Geometry check sheet. Reference: the model listing, model coordinates, mm. Face numbers are marked on the shaded views. A direction names the side the tool comes from. Coordinates: 2 decimals unless noted, no trailing zeros. Write each loop counter-clockwise with the first axis right and the second up, starting at its lowest first coordinate (ties: lowest second). Pieces come first, ordered by that corner, then holes. Notation, with made-up numbers: (-7, 62.5) -> (3, 62.5) arc R20 ccw to (3, 71.5) -> close; hole circle Ø3 at (-7, -18). An arc over 180 degrees is marked (long way). Use a Markdown table: item, result.
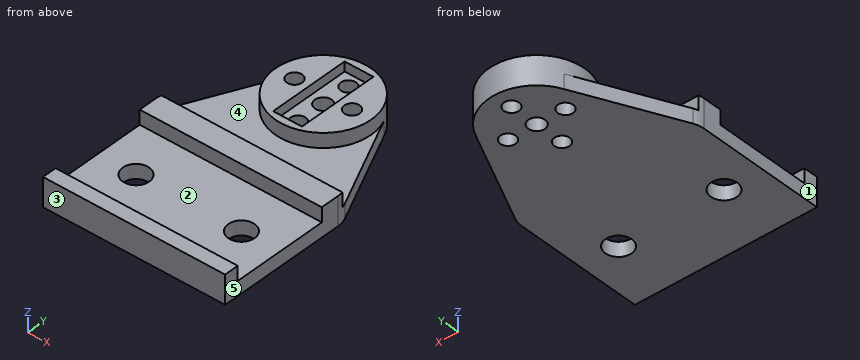
Autodesk Inventor part; units mm, degrees
ref_plane "YZ Plane" through (0, 0, 0) normal (1, 0, 0) x (0, 1, 0)
ref_plane "XZ Plane" through (0, 0, 0) normal (0, 1, 0) x (-1, 0, 0)
ref_plane "XY Plane" through (0, 0, 0) normal (0, 0, 1) x (1, 0, 0)
sketch "スケッチ1" plane through (0, 0, 0) normal (0, 0, 1) x (1, 0, 0)
  line L0 (0, 0) -> (38, 0)
  line L1 (38, 0) -> (38, 28)
  line L2 (0, 28) -> (0, 0)
  circle A0 centre (19, 45) radius 10
  line L3 (19, 45) -> (19, 0)
  line L4 (9, 45) -> (29, 45)
  line L5 (10.069714, 49.5) -> (27.930286, 49.5)
  line L6 (10.069714, 49.5) -> (0, 28)
  line L7 (27.930286, 49.5) -> (38, 28)
  point P0 (28.174131, 48.979363)
  point P1 (9.825869, 48.979363)
  dimension "d0" = 38
  dimension "d1" = 28
  dimension "d3" = 20
  dimension "d56" = 45
  dimension "d71" = 28
  dimension "d73" = 4.5
sketch "スケッチ1 outline for 押し出し1" plane through (0, 0, 0) normal (0, 0, 1) x (1, 0, 0)
  line L0 (9.825869, 48.979363) -> (0, 28)
  line L1 (0, 28) -> (0, 0)
  line L2 (0, 0) -> (38, 0)
  line L3 (38, 0) -> (38, 28)
  line L4 (38, 28) -> (28.174131, 48.979363)
  arc A0 (28.174131, 48.979363) -> (9.825869, 48.979363) centre (19, 45) ccw
extrude "押し出し1" add sketch "スケッチ1 outline for 押し出し1" along normal blind 3
sketch "スケッチ7" plane through (0, 0, 3) normal (0, 0, 1) x (1, 0, 0)
  line L0 (0, 0) -> (38, 0)
  line L1 (38, 0) -> (38, 28)
  line L2 (0, 0) -> (38, 0)
  line L3 (38, 0) -> (38, 3)
  line L4 (38, 3) -> (0, 3)
  line L5 (0, 3) -> (0, 0)
  arc A0 (28.174131, 48.979363) -> (9.825869, 48.979363) centre (19, 45) ccw
  circle A1 centre (19, 45) radius 10
  line L6 (0, 28) -> (0, 0)
  line L7 (0, 28) -> (38, 28)
  line L8 (38, 28) -> (38, 23)
  line L9 (38, 23) -> (0, 23)
  line L10 (0, 23) -> (0, 28)
  point P0 (27.930286, 47.5)
  point P1 (10.069714, 47.5)
  point P2 (0, 23)
  point P3 (29, 43)
  point P4 (9, 43)
  point P5 (10.069714, 47.5)
  point P6 (27.930286, 47.5)
  point P7 (9.486338, 51.080624)
  point P8 (28.513662, 51.080624)
  dimension "d58" = 3
  dimension "d68" = 20
  dimension "d69" = 20
  dimension "d70" = 5
extrude "押し出し4" add sketch "スケッチ7" along normal blind 3 contours L5 L4 L1 L0 | L6 L7 L1 L9 | A1 A0
sketch "スケッチ10" plane through (19, 45, 6) normal (0, 0, 1) x (1, 0, 0)
  line L0 (-3, 8.5) -> (3, 8.5)
  line L1 (3, 8.5) -> (3, -8.5)
  line L2 (3, -8.5) -> (-3, -8.5)
  line L3 (-3, -8.5) -> (-3, 8.5)
  circle A0 centre (0, 0) radius 10
  point P0 (-19, -45)
  dimension "d74" = 8.5
  dimension "d75" = 17
  dimension "d76" = 6
  dimension "d77" = 3
extrude "押し出し7" cut sketch "スケッチ10" against normal blind 2 contours L0 L1 L2 L3
sketch "スケッチ11" plane through (0, 0, 0) normal (0, 0, -1) x (-1, 0, 0)
  arc A0 (-9.825869, 48.979363) -> (-28.174131, 48.979363) centre (-19, 45) ccw
  point P0 (0, 0)
  point P1 (-27.930286, 47.5)
  point P2 (-10.069714, 47.5)
  point P3 (-19, 51)
  point P4 (-25, 45)
  point P5 (-19, 39)
  point P6 (-13, 45)
  dimension "d80" = 6
  dimension "d83" = 360
hole "穴4" at (19, 51, 0) at (25, 45, 0) at (19, 39, 0) at (13, 45, 0) direction (0, 0, 1) diameter 3.2 end through all
sketch "スケッチ12" plane through (0, 0, 0) normal (0, 0, -1) x (-1, 0, 0)
  circle A0 centre (-19, 45) radius 10
  point P0 (0, 0)
hole "穴5" at (19, 45, 0) direction (0, 0, 1) diameter 3.5 end through all
sketch "スケッチ13" plane through (0, 0, 0) normal (0, 0, -1) x (-1, 0, 0)
  circle A0 centre (-19, 45) radius 1.75
  circle A1 centre (-13, 45) radius 1.6
  circle A2 centre (-19, 39) radius 1.6
  circle A3 centre (-25, 45) radius 1.6
  circle A4 centre (-19, 51) radius 1.6
  arc A5 (-9.825869, 48.979363) -> (-28.174131, 48.979363) centre (-19, 45) ccw
  line L0 (-38, 28) -> (-28.174131, 48.979363)
  line L1 (-38, 0) -> (-38, 28)
  line L2 (0, 0) -> (-38, 0)
  line L3 (0, 28) -> (0, 0)
  line L4 (-9.825869, 48.979363) -> (0, 28)
fillet "フィレット1" radius 5 2 edges at (0, 28, 1.5) (38, 28, 1.5)
sketch "スケッチ14" plane through (0, 0, 3) normal (0, 0, 1) x (1, 0, 0)
  line L0 (0, 0) -> (38, 0)
  line L1 (0, 23) -> (0, 3)
  line L2 (38, 3) -> (38, 23)
  point P0 (8, 13)
  point P1 (30, 13)
  dimension "d100" = 13
  dimension "d101" = 13
  dimension "d102" = 8
  dimension "d103" = 8
hole "穴6" at (8, 13, 3) at (30, 13, 3) direction (0, 0, -1) diameter 5.5 end through all
properties part number "robot-arm-frame-base"
Item 1: Section check D-D on x = 19. Record the boundary of the cut face in (y, z), then the cut area to 3 significant figures.
Answer block:
| item | result |
|---|---|
| outline | (0, 0) -> (37.4, 0) -> (37.4, 4) -> (36.5, 4) -> (36.5, 6) -> (35, 6) -> (35, 3) -> (28, 3) -> (28, 6) -> (23, 6) -> (23, 3) -> (3, 3) -> (3, 6) -> (0, 6) -> close; (40.6, 0) -> (43.25, 0) -> (43.25, 4) -> (40.6, 4) -> close; (46.75, 0) -> (49.4, 0) -> (49.4, 4) -> (46.75, 4) -> close; (52.6, 0) -> (55, 0) -> (55, 6) -> (53.5, 6) -> (53.5, 4) -> (52.6, 4) -> close |
| area | 175 mm^2 |
Item 2: Section check C-C on z = 2. Record the boundary of the cut face in (x, y), then the cut area to 3 significant figures.
Answer block:
| item | result |
|---|---|
| outline | (0, 0) -> (38, 0) -> (38, 26.89) arc R5 ccw to (37.53, 29.01) -> (28.17, 48.98) arc R10 ccw to (9.83, 48.98) -> (0.47, 29.01) arc R5 ccw to (0, 26.89) -> close; hole circle Ø5.5 at (8, 13); hole circle Ø3.2 at (13, 45); hole circle Ø3.5 at (19, 45); hole circle Ø3.2 at (19, 39); hole circle Ø3.2 at (19, 51); hole circle Ø3.2 at (25, 45); hole circle Ø5.5 at (30, 13) |
| area | 1,650 mm^2 |
Item 3: Section check A-A on y = 51. Record the boundary of the cut face in (x, z).
Answer block:
| item | result |
|---|---|
| outline | (11, 0) -> (17.4, 0) -> (17.4, 4) -> (16, 4) -> (16, 6) -> (11, 6) -> close; (20.6, 0) -> (27, 0) -> (27, 6) -> (22, 6) -> (22, 4) -> (20.6, 4) -> close |
Item 4: Tool access check on the marked faces 4 and 5. Record the directions out of +Z, -Z, +X, -X, +Y, -Y that give a thin tool (end or side, any length) a straight path to the whole face; none if there is none.
Answer block:
| item | result |
|---|---|
| face 4 | +Z |
| face 5 | +Z, -Z, +X, +Y, -Y |
Item 5: Depth check by flat-ended pin: P1, Ø3.5, axis at x = 19, y = 39, coming from the -Z side; P2, Ø3, axis at x = 33, y = 31, coming from the +Z side; P3, Ø1.5, axis at x = 15.5, z = 5, coming from the +Y side; P4, Ø2.5, axis at x = 27.5, z = 4, coming from the +Y side. Enter the tip coordinate at first touch or a pass-through.
Answer block:
| item | result |
|---|---|
| P1 | stops at z = 0 |
| P2 | stops at z = 3 |
| P3 | stops at y = 54.61 |
| P4 | stops at y = 51.89 |
Item 6: Thickness scan on L1, parallel to X at y = 13, z = 0.9; L2, parallel to Y at x = 19, z = 0.8; L3, parallel to X at y = 45, z = 3.05. Record the ranges inside material, lowest first. Write a range as [from, to].
Answer block:
| item | result |
|---|---|
| L1 | x = [0, 5.25], [10.75, 27.25], [32.75, 38] |
| L2 | y = [0, 37.4], [40.6, 43.25], [46.75, 49.4], [52.6, 55] |
| L3 | x = [9, 11.4], [14.6, 17.25], [20.75, 23.4], [26.6, 29] |
Item 7: Mould release check, pull along Y, two halves, no side actions. Record for the marked faces 1, 2 and 3: +Y half, -Y half, draft (parallel to the pull), parting line (faces both ways), or undercut.
Answer block:
| item | result |
|---|---|
| face 1 | draft |
| face 2 | undercut |
| face 3 | -Y half |
Item 8: Section check B-B on x = 13. Record the boundary of the cut face in (y, z).
Answer block:
| item | result |
|---|---|
| outline | (0, 0) -> (43.4, 0) -> (43.4, 6) -> (37, 6) -> (37, 3) -> (28, 3) -> (28, 6) -> (23, 6) -> (23, 3) -> (3, 3) -> (3, 6) -> (0, 6) -> close; (46.6, 0) -> (53, 0) -> (53, 6) -> (46.6, 6) -> close |
